from build123d import *

# Parameters (mm, degrees)
SKETCH1_W           = 13
SKETCH1_H           = 19
BOSS_EXTRUDE1_DEPTH = 7
SKETCH2_W           = 7
SKETCH2_H           = 0.75
SKETCH2_W_2         = 0.75
SKETCH2_H_2         = 7
SKETCH2_W_3         = 6.972272669
BOSS_EXTRUDE2_DEPTH = 0.2


with BuildPart() as part:
    # Sketch1 → Boss-Extrude1 (new body)
    with BuildSketch(Plane(origin=(0, 0, 0), x_dir=(1, 0, 0), z_dir=(0, 1, 0))):
        with Locations((6.5, -9.363530646)):
            Rectangle(SKETCH1_W, SKETCH1_H)
    extrude(amount=BOSS_EXTRUDE1_DEPTH)

    # Sketch2 → Boss-Extrude2 (add)
    with BuildSketch(Plane(origin=(0, 7, 0), x_dir=(1, 0, 0), z_dir=(0, 1, 0))):
        with Locations((6.722702143, -2.238530646)):
            Rectangle(SKETCH2_W, SKETCH2_H)
        with Locations((2.347702143, -5.363530646)):
            Rectangle(SKETCH2_W_2, SKETCH2_H_2)
        with Locations((11.003251179, -5.363530646)):
            Rectangle(SKETCH2_W_2, SKETCH2_H_2)
        with Locations((6.722702143, -9.488530646)):
            Rectangle(SKETCH2_W, SKETCH2_H)
        with Locations((2.347702143, -13.363530646)):
            Rectangle(SKETCH2_W_2, SKETCH2_H_2)
        with Locations((6.708838478, -17.130647723)):
            Rectangle(SKETCH2_W_3, SKETCH2_H)
        with Locations((11.047702143, -13.363530646)):
            Rectangle(SKETCH2_W_2, SKETCH2_H_2)
    extrude(amount=BOSS_EXTRUDE2_DEPTH)


solid = part.part
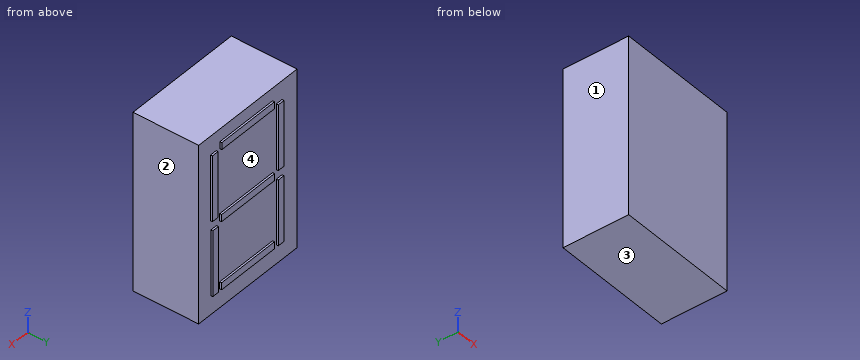
Can you work these out from the model? Positions are in its coordinate system, mm. Face numbers are marked on the shaded views. Give positions to 0.01 mm unless a question says otherwise; leave off trailing zeros. Order: outer loops, then holes, each group sorted by start corner. A loop starts at its lowest first (then second) coordinate and runs counter-clockwise, first axis right, second up. Notation, with made-up numbers: M 38,15.5 L 45,15.5 A22 cw 45,45.5 Z; hole C -38.5,40.5 d11. An arc over 180 degrees is marked long. Use one line per item in the form item = value.
Item 1: Will this pin go through, and if not, where does the flat tip stop? pin 1 Ø2 at (x, z) = (8, 5.5) entering from +Y.
Values follow:
pin_1 = 7
Item 2: If we section it at C-C, the plane x = 1: Write out the boundary of the cut face in (y, z), and give its area (3 significant figures).
Values follow:
outline = M 0,-0.14 L 7,-0.14 L 7,18.86 L 0,18.86 Z
area = 133 mm^2
Item 3: If I drill on line 1 along Y through (x, z) = (9, 13.5), over which ranges is the centre line in solid material (lowest first)? Write a range as [from, to].
Values follow:
line_1 = [0, 7]
Item 4: If we section it at A-A, the plane x = 3.5: Write out the boundary of the cut face in (y, z), and give its area (3 significant figures).
Values follow:
outline = M 0,-0.14 L 7,-0.14 L 7,1.86 L 7.2,1.86 L 7.2,2.61 L 7,2.61 L 7,9.11 L 7.2,9.11 L 7.2,9.86 L 7,9.86 L 7,16.76 L 7.2,16.76 L 7.2,17.51 L 7,17.51 L 7,18.86 L 0,18.86 Z
area = 133 mm^2
Item 5: If we section it at B-B, the plane z = 8: Write out the boundary of the cut face in (x, y), and give its area (3 significant figures).
Values follow:
outline = M 0,0 L 13,0 L 13,7 L 11.38,7 L 11.38,7.2 L 10.63,7.2 L 10.63,7 L 2.72,7 L 2.72,7.2 L 1.97,7.2 L 1.97,7 L 0,7 Z
area = 91.3 mm^2
Item 6: Thinking about a two-plate mould opening in X: for the marked faces 1, 2, 3 and 4, which applies, pulls with the +X half, pulls with the -X half, needs draft (parallel to the pull), parting line crosses it, or undercut?
Values follow:
face_1 = pulls with the -X half
face_2 = pulls with the +X half
face_3 = needs draft
face_4 = undercut
